Can you work these out from the model? Positions are in its coordinate system, mm. Round coordinates to 2 decimals unless told otherwise and drop trailing zeros. Loops run counter-clockwise (first coordinate to the right, second up) from the corner with the lowest first, then second, coordinate; pieces in that order, holes last. Notation, with made-up numbers: (1.25, -22) -> (20.25, -22) arc R28 ccw to (20.25, 12) -> close; hole circle Ø8 at (14, 49). An arc over 180 degrees is marked (long way). Use a Markdown table: item, result.
Autodesk Inventor part; units mm, degrees
ref_plane "YZ Plane" through (0, 0, 0) normal (1, 0, 0) x (0, 1, 0)
ref_plane "XZ Plane" through (0, 0, 0) normal (0, 1, 0) x (-1, 0, 0)
ref_plane "XY Plane" through (0, 0, 0) normal (0, 0, 1) x (1, 0, 0)
sketch "Sketch1" plane through (0, 0, 0) normal (0, 1, 0) x (-1, 0, 0)
  line L0 (0, 0) -> (35, 0)
  line L1 (35, 0) -> (35, -40)
  line L2 (35, -40) -> (0, -40)
  line L3 (0, -40) -> (0, 0)
  line L4 (35, -40) -> (0, 0) construction
  line L5 (35, 0) -> (0, -40) construction
  line L6 (4.5, -5) -> (30.5, -5) construction
  line L7 (30.5, -5) -> (30.5, -35) construction
  line L8 (30.5, -35) -> (4.5, -35) construction
  line L9 (4.5, -35) -> (4.5, -5) construction
  line L10 (4.5, -5) -> (30.5, -35) construction
  line L11 (30.5, -5) -> (4.5, -35) construction
  circle A0 centre (30.5, -5) radius 2.5
  circle A1 centre (30.5, -35) radius 2.5
  circle A2 centre (4.5, -35) radius 2.5
  circle A3 centre (4.5, -5) radius 2.5
  point P0 (17.5, -20)
  dimension "d0" = 35
  dimension "d1" = 40
  dimension "d2" = 26
  dimension "d3" = 30
  dimension "d4" = 5
extrude "Extrusion1" add sketch "Sketch1" along normal blind 2
sketch "Sketch3" plane through (0, 0, 0) normal (0, -1, 0) x (1, 0, 0)
  line L0 (-35, 0) -> (0, -40) construction
  line L1 (0, 0) -> (-35, -40) construction
  circle A0 centre (-12.232, -13.9794) radius 1
  point P0 (-17.5, -20)
  point P1 (-17.5, -20)
  dimension "d19" = 2
  dimension "d20" = 8
extrude "Extrusion2" cut sketch "Sketch3" against normal blind 10
pattern_circular "Circular Pattern1" count 3 over 360 about axis through (-17.5, 0, -20) along (0, -1, 0) of "Extrusion2"
properties part number "carbon_bump_gimbal"
1. I need wall thicknesses on line 1 (Z direction, x = -30.5, y = 0.6); line 2 (X direction, y = 1.05, z = -6.5); line 3 (Z direction, x = -31, y = 1). Which ranges of each line are inside material? Lowest first, please.
Answer sheet:
| item | result |
|---|---|
| line 1 | z = -40 to -37.5, -32.5 to -7.5, -2.5 to 0 |
| line 2 | x = -35 to -32.5, -28.5 to -6.5, -2.5 to 0 |
| line 3 | z = -40 to -37.45, -32.55 to -7.45, -2.55 to 0 |
2. I want a section at D-D (y = 0.95). Please give me the cut outline in (x, z).
Answer sheet:
| item | result |
|---|---|
| outline | (-35, -40) -> (0, -40) -> (0, 0) -> (-35, 0) -> close; hole circle Ø5 at (-30.5, -35); hole circle Ø5 at (-30.5, -5); hole circle Ø2 at (-25.35, -18.45); hole circle Ø2 at (-14.92, -27.57); hole circle Ø2 at (-12.23, -13.98); hole circle Ø5 at (-4.5, -35); hole circle Ø5 at (-4.5, -5) |
3. If we mould it in two halves opening along Z, with no side actions, what happens to faces 1 (the flat face through (-17, 0, -20)), 2 (the flat face through (-17, 1, 0)), 3 (the cylindrical face through (-6.885, 0.986, -35.751))? For each: +Z half, -Z half, draft (parallel to the pull), parting line (faces both ways), or undercut.
Answer sheet:
| item | result |
|---|---|
| face 1 | draft |
| face 2 | +Z half |
| face 3 | undercut |
4. I want a section at C-C (x = -25). Please give me the cut outline in (y, z).
Answer sheet:
| item | result |
|---|---|
| outline | (0, -40) -> (2, -40) -> (2, -19.39) -> (0, -19.39) -> close; (0, -17.51) -> (2, -17.51) -> (2, 0) -> (0, 0) -> close |
5. I want a section at B-B (z = -5). Please give me the cut outline in (x, y).
Answer sheet:
| item | result |
|---|---|
| outline | (-35, 0) -> (-33, 0) -> (-33, 2) -> (-35, 2) -> close; (-28, 0) -> (-7, 0) -> (-7, 2) -> (-28, 2) -> close; (-2, 0) -> (0, 0) -> (0, 2) -> (-2, 2) -> close |
6. I want a section at A-A (x = -29). Please give me the cut outline in (y, z), plus the area to 3 significant figures.
Answer sheet:
| item | result |
|---|---|
| outline | (0, -40) -> (2, -40) -> (2, -37) -> (0, -37) -> close; (0, -33) -> (2, -33) -> (2, -7) -> (0, -7) -> close; (0, -3) -> (2, -3) -> (2, 0) -> (0, 0) -> close |
| area | 64.0 mm² |
